Check sheet for the modelled part. Datum: model origin and axes. Units: mm. A direction names the side the tool comes from. Round coordinates to 2 decimals unless told otherwise and drop trailing zeros. Put each result on its own line as item: value.
```python
from build123d import *

# Parameters (mm, degrees)
SKETCH1_R               = 40
BOSS_EXTRUDE1_DEPTH     = 74.5
SKETCH3_R               = 40
SKETCH3_R_2             = 25
CUT_EXTRUDE1_DEPTH      = 21
CUT_EXTRUDE2_DEPTH      = 22
CUT_EXTRUDE2_DEPTH_BACK = 22
SKETCH2_R               = 40
SKETCH2_R_2             = 37.5
CUT_EXTRUDE4_DEPTH      = 160.376911753
FILLET1_R               = 2
CUT_EXTRUDE5_DEPTH      = 160.376911753
SKETCH8_R               = 3.75
CUT_EXTRUDE6_DEPTH      = 140.942845476
CUT_EXTRUDE7_DEPTH      = 94.542770966


with BuildPart() as part:
    # Sketch1 → Boss-Extrude1 (new, symmetric)
    with BuildSketch(Plane(origin=(0, 0, 0), x_dir=(1, 0, 0), z_dir=(0, 1, 0))):
        with Locations(Location((0, 0, 0), (0, 0, 270))):
            Circle(SKETCH1_R)
    extrude(amount=BOSS_EXTRUDE1_DEPTH, both=True)

    # Sketch3 → Cut-Extrude1 (cut)
    with BuildSketch(Plane(origin=(0, 74.5, 0), x_dir=(1, 0, 0), z_dir=(0, 1, 0))):
        with Locations(Location((0, 0, 0), (0, 0, 270))):
            Circle(SKETCH3_R)
        with Locations(Location((0, 0, 0), (0, 0, 270))):
            Circle(SKETCH3_R_2, mode=Mode.SUBTRACT)
    cut_extrude1 = extrude(amount=-CUT_EXTRUDE1_DEPTH, mode=Mode.SUBTRACT)

    # Mirror1: Cut-Extrude1 across plane
    add(cut_extrude1.mirror(Plane.ZX), mode=Mode.SUBTRACT)

    # Sketch2 → Cut-Extrude2 (cut, two sides: drawn at the far end of the back side and taken through both)
    with BuildSketch(Plane(origin=(0, 0, 0), x_dir=(1, 0, 0), z_dir=(0, 1, 0)).offset(-CUT_EXTRUDE2_DEPTH_BACK)):
        with Locations(Location((0, 0, 0), (0, 0, 270))):
            Circle(SKETCH2_R)
        with Locations(Location((0, 0, 0), (0, 0, 90))):
            Circle(SKETCH2_R_2, mode=Mode.SUBTRACT)
    extrude(amount=CUT_EXTRUDE2_DEPTH + CUT_EXTRUDE2_DEPTH_BACK, mode=Mode.SUBTRACT)

    # Sketch5 → Cut-Extrude4 (cut, through all)
    with BuildSketch(Plane(origin=(0, 74.5, 0), x_dir=(1, 0, 0), z_dir=(0, 1, 0))):
        with BuildLine():
            Line((-12, 13), (12, 13))
            ThreePointArc((12, 13), (15, 10), (12, 7))
            Line((12, 7), (-12, 7))
            ThreePointArc((-12, 7), (-15, 10), (-12, 13))
        make_face()
    extrude(amount=-CUT_EXTRUDE4_DEPTH, mode=Mode.SUBTRACT)

    # Fillet1
    fillet1_edges = [part.edges().sort_by_distance(p)[0] for p in [
        (0, -53.5, -25),
        (0, 53.5, -25),
    ]]
    fillet(fillet1_edges, radius=FILLET1_R)

    # Sketch7 → Revolve2 (revolve)
    with BuildSketch(Plane(origin=(0, 0, 0), x_dir=(0, 0, -1), z_dir=(1, 0, 0))):
        Polygon((40, 22), (37.5, 19.5), (37.5, 22), align=None)
    revolve2 = revolve(axis=Axis((0, 103.881416882, 0), (0, -1, 0)))

    # Mirror2: Revolve2 across plane
    add(revolve2.mirror(Plane.ZX))

    # Sketch4 → Cut-Extrude5 (cut, through all)
    with BuildSketch(Plane(origin=(0, 74.5, 0), x_dir=(1, 0, 0), z_dir=(0, 1, 0))):
        with BuildLine():
            Line((0, 0), (0, 40))
            ThreePointArc((0, 40), (28.284271247, 28.284271247), (40, 0))
            Line((40, 0), (0, 0))
        make_face()
    extrude(amount=-CUT_EXTRUDE5_DEPTH, mode=Mode.SUBTRACT)

    # Sketch8 → Cut-Extrude6 (cut, through all)
    with BuildSketch(Plane(origin=(0, 53.5, 0), x_dir=(1, 0, 0), z_dir=(0, 1, 0))):
        with Locations(Location((-8.282209443, 30.909626441, 0), (0, 0, 270))):
            Circle(SKETCH8_R)
        with Locations(Location((30.909626441, -8.282209443, 0), (0, 0, 270))):
            Circle(SKETCH8_R)
        with Locations(Location((22.627416998, -22.627416998, 0), (0, 0, 270))):
            Circle(SKETCH8_R)
        with Locations(Location((8.282209443, -30.909626441, 0), (0, 0, 270))):
            Circle(SKETCH8_R)
        with Locations(Location((-8.282209443, -30.909626441, 0), (0, 0, 270))):
            Circle(SKETCH8_R)
        with Locations(Location((-22.627416998, -22.627416998, 0), (0, 0, 270))):
            Circle(SKETCH8_R)
        with Locations(Location((-30.909626441, -8.282209443, 0), (0, 0, 270))):
            Circle(SKETCH8_R)
        with Locations(Location((-30.909626441, 8.282209443, 0), (0, 0, 270))):
            Circle(SKETCH8_R)
        with Locations(Location((-22.627416998, 22.627416998, 0), (0, 0, 270))):
            Circle(SKETCH8_R)
    extrude(amount=-CUT_EXTRUDE6_DEPTH, mode=Mode.SUBTRACT)

    # Sketch10 → Cut-Extrude7 (cut, through all)
    with BuildSketch(Plane(origin=(0, 0, 0), x_dir=(-1, 0, 0), z_dir=(0, 0, -1))):
        with BuildLine():
            Line((-25.208360839, -42.779227454), (-27.321452148, -47.310766389))
            ThreePointArc((-27.321452148, -47.310766389), (-33.506811582, -45.211119786), (-40, -44.5))
            Line((-40, -44.5), (-40, -53.5))
            Line((-40, -53.5), (-27, -53.5))
            ThreePointArc((-27, -53.5), (-25.585786438, -54.085786438), (-25, -55.5))
            Line((-25, -55.5), (-25, -74.5))
            Line((-25, -74.5), (-10, -74.5))
            ThreePointArc((-10, -74.5), (-10.114159057, -71.885327718), (-10.45576741, -69.29055467))
            Line((-10.45576741, -69.29055467), (-5.531728645, -68.422313782))
            ThreePointArc((-5.531728645, -68.422313782), (-12.23263309, -53.193349985), (-25.208360839, -42.779227454))
        make_face()
    extrude(amount=-CUT_EXTRUDE7_DEPTH, mode=Mode.SUBTRACT)


solid = part.part
```
1. Access from +Z, -Z, +X, -X, +Y, -Y to the whole of each face (thin tool, end or side, straight path). Record for faces 5 (the flat face through (0, 1, -26)), 6 (the flat face through (-6, 1, -13)), 7 (the conical face through (-25.711, 19.621, 27.465)), 8 (the flat face through (8.028, -68.863, 12.019)), 9 (the flat face through (26.25, -45.01, 15.31)).
Computed values:
face 5: -Z, +X, +Y, -Y
face 6: +X, +Y, -Y
face 7: none
face 8: +Z, -Z, +X
face 9: +Z, -Z, -Y
2. Depth check by flat-ended pin: pin 1 Ø4 at (x, y) = (-15, -18.5) entering from -Z; pin 2 Ø6 at (x, y) = (-4, 5.5) entering from +Z; pin 3 Ø1.5 at (x, z) = (-5.5, -27) entering from -Y; pin 4 Ø7 at (x, z) = (-30.91, 8.28) entering from +Y. Enter the tip coordinate at first touch or a pass-through.
Computed values:
pin 1: stops at z = -35.61
pin 2: stops at z = 37.49
pin 3: stops at y = -53.51
pin 4: passes through
3. Cross-section at A-A (y = 41.5). Count the separate pieces of the cut face and the enclosed holes in it, then the cut area to 3 significant figures.
Computed values:
separate pieces: 1
enclosed holes: 9
area: 3,290 mm2
4. Scan lines: probe 1 along X at (y, z) = (46.5, 33.5); probe 2 along Z at (x, y) = (-28.5, -47); probe 3 along X at (y, z) = (-24, 8). Record each from-to range of solid material in increasing order.
Computed values:
probe 1: x = -21.86 to -10.99, -5.57 to 5.57, 10.99 to 21.86
probe 2: z = -28.07 to -11.16, -5.41 to 5.41, 11.16 to 28.07
probe 3: x = -39.19 to -34.65, -27.17 to 27.17, 34.65 to 39.19
5. Release check for a two-part mould opening along X. For faces 1 (the conical face through (-25.711, -19.621, 27.465)), 2 (the cylindrical face through (-15, 1, -10)), 3 (the cylindrical face through (-11.943, 0.749, -31.723)), 4 (the cylindrical face through (-29.8, 0.7, -4.7)) record: +X half, -X half, draft (parallel to the pull), parting line (faces both ways), or undercut.
Computed values:
face 1: parting line
face 2: +X half
face 3: undercut
face 4: undercut
